Could you check a few things on this drawing? It's one solid part, dimensions in mm from its lowest x, y, z. A direction names the side the tool comes from. Round coordinates to 2 decimals unless told otherwise and drop trailing zeros. Loops run counter-clockwise (first coordinate to the right, second up) from the corner with the lowest first, then second, coordinate; pieces in that order, holes last. Notation, with made-up numbers: (73.25, 34) -> (88.25, 34) arc R27 ccw to (88.25, 54) -> close; hole circle Ø4 at (-7.5, -12). An arc over 180 degrees is marked (long way). Write each question's results on one line, items separated by ' | '.
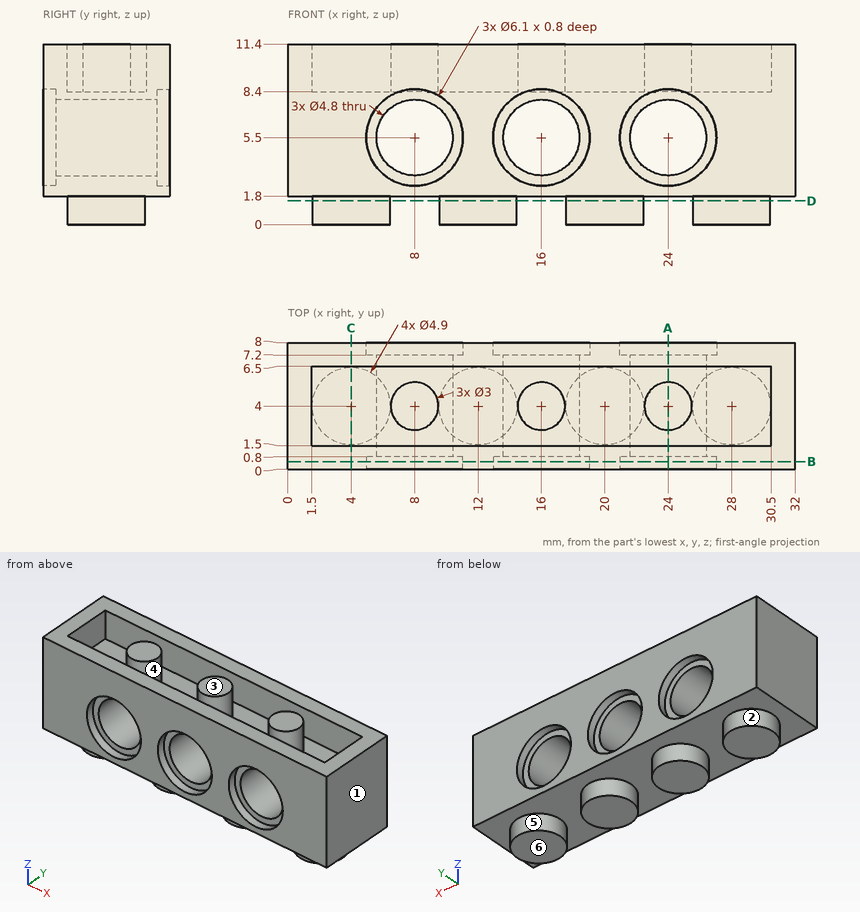
1) I need wall thicknesses on line 1 (X direction, y = 5.25, z = 10.25); line 2 (X direction, y = 3.75, z = 9.75); line 3 (Y direction, x = 3, z = 9.75). Which ranges of each line are inside material? Lowest first, please.
Model answer:
line 1: x = 0 to 1.5, 7.17 to 8.83, 15.17 to 16.83, 23.17 to 24.83, 30.5 to 32 | line 2: x = 0 to 1.5, 6.52 to 9.48, 14.52 to 17.48, 22.52 to 25.48, 30.5 to 32 | line 3: y = 0 to 1.5, 6.5 to 8
2) If we mould it in two halves opening along X, with no side actions, what happens to the marked faces 1, 2 and 3? For each: released by +X, released by -X, zero draft, split by the parting line, or undercut.
Model answer:
face 1: released by +X | face 2: undercut | face 3: zero draft
3) I want a section at C-C, the plane x = 4. Write out the boundary of the cut face in (y, z), plus the area to 3 significant figures.
Model answer:
outline: (0, 1.8) -> (1.55, 1.8) -> (1.55, 0) -> (6.45, 0) -> (6.45, 1.8) -> (8, 1.8) -> (8, 11.4) -> (6.5, 11.4) -> (6.5, 8.4) -> (1.5, 8.4) -> (1.5, 11.4) -> (0, 11.4) -> close | area: 70.6 mm2
4) I want a section at A-A, the plane x = 24. Write out the boundary of the cut face in (y, z), plus the area to 3 significant figures.
Model answer:
outline: (0, 1.8) -> (8, 1.8) -> (8, 2.45) -> (7.2, 2.45) -> (7.2, 3.1) -> (0.8, 3.1) -> (0.8, 2.45) -> (0, 2.45) -> close; (0, 8.55) -> (0.8, 8.55) -> (0.8, 7.9) -> (7.2, 7.9) -> (7.2, 8.55) -> (8, 8.55) -> (8, 11.4) -> (6.5, 11.4) -> (6.5, 8.4) -> (5.5, 8.4) -> (5.5, 11.4) -> (2.5, 11.4) -> (2.5, 8.4) -> (1.5, 8.4) -> (1.5, 11.4) -> (0, 11.4) -> close | area: 30.3 mm2
5) I want a section at B-B, the plane y = 0.5. Write out the boundary of the cut face in (x, z).
Model answer:
outline: (0, 1.8) -> (32, 1.8) -> (32, 11.4) -> (0, 11.4) -> close; hole circle Ø6.1 at (8, 5.5); hole circle Ø6.1 at (16, 5.5); hole circle Ø6.1 at (24, 5.5)
6) For the marked faces 4, 5 and 6, which set-ups out of +Z, -Z, +X, -X, +Y, -Y let a thin tool reach every point of the face, with its end or its side?
Model answer:
face 4: +Z | face 5: -Z | face 6: -Z, +X, -X, +Y, -Y
7) I'm going to push flat-ended pins straight in: pin 1 (5 mm diameter, centred on x = 23.5, z = 5.5, fed in from -Y); pin 2 (3 mm diameter, centred on x = 16, z = 5.5, fed in from +Y); pin 3 (1.5 mm diameter, centred on x = 13.5, z = 10.5, fed in from -Y); pin 4 (2.5 mm diameter, centred on x = 15.5, y = 5.5, fed in from -Z). Where does each tip first touch, or does it pass through?
Model answer:
pin 1: stops at y = 0.8 | pin 2: passes through | pin 3: stops at y = 0 | pin 4: stops at z = 1.8
8) I want a section at D-D, the plane z = 1.5. Write out the boundary of the cut face in (x, y), plus the area to 3 significant figures.
Model answer:
outline: circle Ø4.9 at (4, 4); circle Ø4.9 at (12, 4); circle Ø4.9 at (20, 4); circle Ø4.9 at (28, 4) | area: 75.4 mm2
